Autodesk Inventor part; units mm, degrees
ref_plane "YZ Plane" through (0, 0, 0) normal (1, 0, 0) x (0, 1, 0)
ref_plane "XZ Plane" through (0, 0, 0) normal (0, 1, 0) x (-1, 0, 0)
ref_plane "XY Plane" through (0, 0, 0) normal (0, 0, 1) x (1, 0, 0)
sketch "Sketch1" plane through (0, 0, 0) normal (0, 0, 1) x (1, 0, 0)
  line L0 (0, 0) -> (50, 0)
  line L1 (50, 0) -> (50, 21.8)
  line L2 (50, 21.8) -> (0, 21.8)
  line L3 (0, 21.8) -> (0, 0)
  circle A0 centre (8, 10.9) radius 1.65
  circle A1 centre (32, 10.9) radius 1.65
  line L4 (50, 14.4) -> (43, 14.4)
  line L5 (43, 14.4) -> (43, 7.4)
  line L6 (43, 7.4) -> (50, 7.4)
  line L7 (50, 7.4) -> (50, 14.4)
  point P0 (46.5, 14.4)
  dimension "d0" = 50
  dimension "d1" = 21.8
  dimension "d2" = 3.3
  dimension "d3" = 3.3
  dimension "d4" = 8
  dimension "d5" = 24
  dimension "d6" = 10.9
  dimension "d7" = 10.9
  dimension "d10" = 7
  dimension "d11" = 7
  dimension "d12" = 7.4
extrude "Extrusion1" add sketch "Sketch1" along normal blind 1.6 contours L3 L2 L1 L4 L5 L6 L0
sketch "Sketch2" plane through (0, 0, 0) normal (0, -1, 0) x (1, 0, 0)
  line L0 (50, 0) -> (50, 1.6)
  line L1 (50, 1.6) -> (44, 1.6)
  line L2 (44, 1.6) -> (44, 3.1)
  line L3 (44, 3.1) -> (50, 3.1)
  line L4 (50, 3.1) -> (50, 1.6)
  circle A0 centre (47, 3.6) radius 2
  point P0 (0, 0)
  point P1 (47, 1.6)
  point P2 (47, 1.6)
  point P3 (45.0635, 3.1)
  point P4 (48.9365, 3.1)
  dimension "d13" = 6
  dimension "d14" = 1.5
  dimension "d15" = 4
  dimension "d16" = 2
  dimension "d17" = 3
extrude "Extrusion2" add sketch "Sketch2" against normal blind 21.8 contours L1 A0 L3 L4 | L1 L2 L3 A0
sketch "Sketch3" plane through (0, 0, 1.6) normal (0, 0, 1) x (1, 0, 0)
  line L0 (50, 7.4) -> (50, 14.4)
  line L1 (43, 14.4) -> (50, 14.4)
  line L2 (50, 14.4) -> (50, 7.4)
  line L3 (50, 7.4) -> (43, 7.4)
  line L4 (43, 7.4) -> (43, 14.4)
  point P0 (0, 0)
extrude "Extrusion3" cut sketch "Sketch3" along normal blind 5 and the other way blind 5
properties part number "Counter"
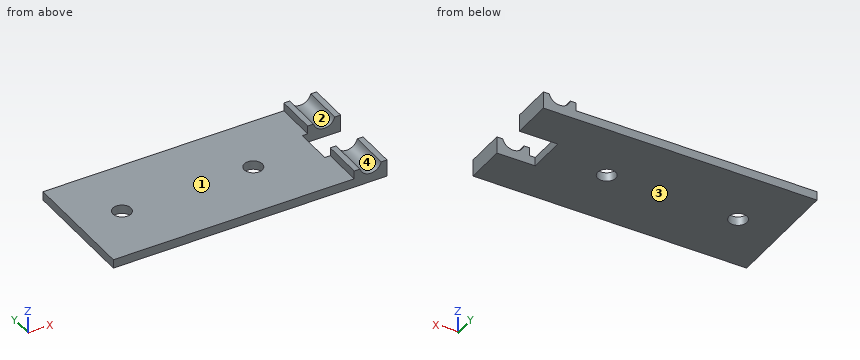
Geometry check sheet. Reference: the model listing, model coordinates, mm. Face numbers are marked on the shaded views. A direction names the side the tool comes from. Give positions to 0.01 mm unless a question says otherwise; leave off trailing zeros. Loops run counter-clockwise (first coordinate to the right, second up) from the corner with the lowest first, then second, coordinate; pieces in that order, holes last. Notation, with made-up numbers: M -23.75,55.5 L -6.75,55.5 A20 cw -6.75,78.5 Z; hole C 0,29.25 d11. An arc over 180 degrees is marked long. Write item = value, one per line.
(1) Sectioned sample at D-D, the plane y = 4.5. Record the cut outline in (x, z).
Answer below:
outline = M 0,0 L 50,0 L 50,3.1 L 48.94,3.1 A2 cw 45.06,3.1 L 44,3.1 L 44,1.6 L 0,1.6 Z
(2) Material ranges on line 1 (Y direction, x = 32, z = 1); line 2 (Z direction, x = 47, y = 2.5); line 3 (X direction, y = 12, z = 0.5), recorded low to high. Write a range as [from, to].
Answer below:
line_1 = [0, 9.25], [12.55, 21.8]
line_2 = [0, 1.6]
line_3 = [0, 6.77], [9.23, 30.77], [33.23, 43]
(3) Gauge pin test, flat ends, axial feed: pin 1 Ø1.2 at (y, z) = (18, 2.5) entering from -X; pin 2 Ø1.3 at (y, z) = (12, 1) entering from +X; pin 3 Ø10 at (x, y) = (30.5, 5) entering from +Z. Record the tip position at first contact, or that the pin passes through.
Answer below:
pin_1 = 44
pin_2 = 43
pin_3 = 1.6
(4) Release check for a two-part mould opening along X. For the marked faces 3 and 4 record: released by +X, released by -X, zero draft, split by the parting line, or undercut.
Answer below:
face_3 = zero draft
face_4 = undercut
(5) Sectioned sample at A-A, the plane x = 32. Record the cut outline in (y, z), plus the area to 3 significant figures.
Answer below:
outline = M 0,0 L 9.25,0 L 9.25,1.6 L 0,1.6 Z; M 12.55,0 L 21.8,0 L 21.8,1.6 L 12.55,1.6 Z
area = 29.6 mm2
(6) Sectioned sample at B-B, the plane y = 10.9. Record the cut outline in (x, z).
Answer below:
outline = M 0,0 L 6.35,0 L 6.35,1.6 L 0,1.6 Z; M 9.65,0 L 30.35,0 L 30.35,1.6 L 9.65,1.6 Z; M 33.65,0 L 43,0 L 43,1.6 L 33.65,1.6 Z
(7) Sectioned sample at C-C, the plane z = 0.65. Record the cut outline in (x, y), plus the area to 3 significant figures.
Answer below:
outline = M 0,0 L 50,0 L 50,7.4 L 43,7.4 L 43,14.4 L 50,14.4 L 50,21.8 L 0,21.8 Z; hole C 8,10.9 d3.3; hole C 32,10.9 d3.3
area = 1,020 mm2
(8) Tool access check on the marked faces 1 and 2. Record the directions out of +Z, -Z, +X, -X, +Y, -Y that give a thin tool (end or side, any length) a straight path to the whole face; none if there is none.
Answer below:
face_1 = +Z, -X, +Y, -Y
face_2 = +Z, +Y, -Y
